Source: CAD feature listing. Evaluate the final solid. Frame: model axes, mm. Face numbers are marked on the shaded views. A direction names the side the tool comes from. Give positions to 0.01 mm unless a question says otherwise; leave off trailing zeros. Order: outer loops, then holes, each group sorted by start corner. A loop starts at its lowest first (then second) coordinate and runs counter-clockwise, first axis right, second up. Notation, with made-up numbers: M -9,69.25 L 38,69.25 A15 cw 38,84.25 Z; hole C 66,-38.5 d9. An arc over 180 degrees is marked long. Answer as a JSON object with one key per item and string values. Group by question number.
1. Section query D-D (x = -21). Output: boundary loops of the cut face in (y, z), plus the area to 3 significant figures.
2. Set-up query: the marked faces 4, 5 and 6. Return all of +Z, -Z, +X, -X, +Y, -Y with unobstructed straight access to the full face (end or side cutting, diameter ignored); none if empty.
3. Section query C-C (z = 5.25). Output: boundary loops of the cut face in (x, y), plus the area to 3 significant figures.
4. Pin query (flat end, axial travel): P1, Ø1.5, axis at x = -25.5, y = -0.5, coming from the +Z side; P2, Ø2, axis at x = 10.5, z = 3.5, coming from the -Y side; P3, Ø15.5, axis at x = 12, y = -11, coming from the -Z side; P4, Ø4.5, axis at x = 11.5, y = 17.5, coming from the +Z side. Return the tip coordinate at first contact, or that it passes through.
5. Pull-direction query (Y, two-part tool) for the marked faces 1, 2 and 3; classes: +Y half, -Y half, draft (parallel to the pull), parting line (faces both ways), or undercut.
6. Section query B-B (x = 10.5). Output: boundary loops of the cut face in (y, z).
7. Section query A-A (y = 12.5). Output: boundary loops of the cut face in (x, z), plus the area to 3 significant figures.
8. Material intervals for L1, parallel to Y at x = 0, z = -2.5; L2, parallel to X at y = -10, z = -2; L3, parallel to Y at x = 0, z = -4.5, sorted ascending. Write a range as [from, to].
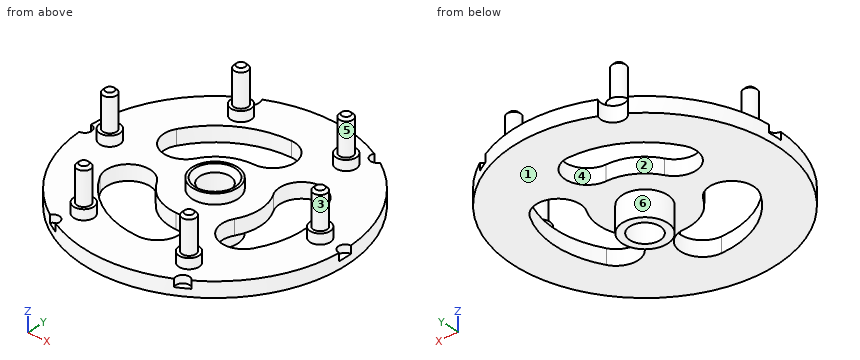
from build123d import *

# Parameters (mm, degrees)
SKETCH_1_R               = 26
EXTRUDE_1_DEPTH          = 3
SKETCH_2_R               = 1.35
EXTRUDE_2_DEPTH          = 9
SKETCH_4_R               = 2
EXTRUDE_4_DEPTH          = 2
SKETCH_5_R               = 3
CUT_EXTRUDE_1_DEPTH      = 38.854986461
SKETCH_7_R               = 4.5
SKETCH_7_R_2             = 3
EXTRUDE_1_2_DEPTH        = 8
EXTRUDE_START            = 2
SKETCH_8_R               = 4.5
SKETCH_8_R_2             = 3
EXTRUDE_2_2_DEPTH        = 2
CUT_EXTRUDE_2_REACH      = 39.855
SKETCH_9_R               = 2.326383569
SKETCH_10_R              = 1.343821969
CUT_EXTRUDE_3_DEPTH      = 1.5
CUT_EXTRUDE_4_REACH      = 40.678
CHAMFER_1_SIZE           = 1
CHAMFER_3_SIZE           = 0.5
PATTERN_CIRCULAR_1_COUNT = 3


with BuildPart() as part:
    # Sketch 1 → Extrude 1 (new body)
    with BuildSketch(Plane.XY):
        Circle(SKETCH_1_R)
    extrude(amount=-EXTRUDE_1_DEPTH)

    # Sketch 2 → Extrude 2 (add)
    with BuildSketch(Plane.XY):
        with Locations((-21, 0)):
            Circle(SKETCH_2_R)
        with Locations((-10.5, 18.186533479)):
            Circle(SKETCH_2_R)
        with Locations((10.5, 18.186533479)):
            Circle(SKETCH_2_R)
        with Locations((21, 0)):
            Circle(SKETCH_2_R)
        with Locations((10.5, -18.186533479)):
            Circle(SKETCH_2_R)
        with Locations((-10.5, -18.186533479)):
            Circle(SKETCH_2_R)
    extrude(amount=EXTRUDE_2_DEPTH)

    # Sketch 4 → Extrude 4 (add)
    with BuildSketch(Plane.XY):
        with Locations((-10.5, 18.186533479)):
            Circle(SKETCH_4_R)
        with Locations((10.5, 18.186533479)):
            Circle(SKETCH_4_R)
        with Locations((21, 0)):
            Circle(SKETCH_4_R)
        with Locations((10.5, -18.186533479)):
            Circle(SKETCH_4_R)
        with Locations((-10.5, -18.186533479)):
            Circle(SKETCH_4_R)
        with Locations((-21, 0)):
            Circle(SKETCH_4_R)
    extrude(amount=EXTRUDE_4_DEPTH)

    # Sketch 5 → Cut-Extrude 1 (cut, through all)
    with BuildSketch(Plane.XY):
        Circle(SKETCH_5_R)
    extrude(amount=-CUT_EXTRUDE_1_DEPTH, mode=Mode.SUBTRACT)

    # Sketch 7 → Extrude 1 2 (add)
    with BuildSketch(Plane.XY):
        Circle(SKETCH_7_R)
        Circle(SKETCH_7_R_2, mode=Mode.SUBTRACT)
    extrude(amount=-EXTRUDE_1_2_DEPTH)

    # Sketch 8 → Extrude 2 2 (add)
    with BuildSketch(Plane.XY.offset(EXTRUDE_START)):
        Circle(SKETCH_8_R)
        Circle(SKETCH_8_R_2, mode=Mode.SUBTRACT)
    extrude(amount=-EXTRUDE_2_2_DEPTH)

    # Sketch 9 → Cut-Extrude 2 (cut, up to next)
    with BuildSketch(Plane.XY, mode=Mode.PRIVATE) as cut_extrude_2_sk1:
        with Locations((-13, 22.516660498)):
            Circle(SKETCH_9_R)
    cut_extrude_2_tool1 = extrude(cut_extrude_2_sk1.sketch, amount=-CUT_EXTRUDE_2_REACH, mode=Mode.PRIVATE) & part.part
    add(cut_extrude_2_tool1.solids().sort_by_distance((-13, 22.51666, 0))[0], mode=Mode.SUBTRACT)

    # Sketch 10 → Cut-Extrude 3 (cut)
    with BuildSketch(Plane.XY):
        with Locations((-13, 22.516660498)):
            Circle(SKETCH_10_R)
        with Locations((13, 22.516660498)):
            Circle(SKETCH_10_R)
        with Locations((26, 0)):
            Circle(SKETCH_10_R)
        with Locations((13, -22.516660498)):
            Circle(SKETCH_10_R)
        with Locations((-13, -22.516660498)):
            Circle(SKETCH_10_R)
        with Locations((-26, 0)):
            Circle(SKETCH_10_R)
    extrude(amount=-CUT_EXTRUDE_3_DEPTH, mode=Mode.SUBTRACT)

    # Sketch 11 → Cut-Extrude 4 (cut, up to next)
    with BuildSketch(Plane(origin=(0, 0, -3), x_dir=(-1, 0, 0), z_dir=(0, 0, -1)), mode=Mode.PRIVATE) as cut_extrude_4_sk1:
        with BuildLine():
            ThreePointArc((15.338641918, 8.855769041), (8.855769041, 15.338641918), (0, 17.711538081))
            ThreePointArc((0, 17.711538081), (-4.370103516, 13.341434566), (0, 8.97133105))
            ThreePointArc((0, 8.97133105), (4.485665525, 7.769400595), (7.769400595, 4.485665525))
            ThreePointArc((7.769400595, 4.485665525), (13.739073015, 2.886096621), (15.338641918, 8.855769041))
        make_face()
    cut_extrude_4_tool1 = extrude(cut_extrude_4_sk1.sketch, amount=-CUT_EXTRUDE_4_REACH, mode=Mode.PRIVATE) & part.part
    cut_extrude_4 = cut_extrude_4_tool1.solids().sort_by_distance((-6.174677, 10.694854, -3))[0]
    add(cut_extrude_4, mode=Mode.SUBTRACT)

    # Chamfer 1
    chamfer_1_edges = [part.edges().sort_by_distance(p)[0] for p in [
        (-3, 0, 2),
    ]]
    chamfer(chamfer_1_edges, length=CHAMFER_1_SIZE)

    # Chamfer 3
    chamfer_3_edges = [part.edges().sort_by_distance(p)[0] for p in [
        (-11.85, 18.186533479, 9),
        (9.15, 18.186533479, 9),
        (19.65, 0, 9),
        (9.15, -18.186533479, 9),
        (-11.85, -18.186533479, 9),
        (-22.35, 0, 9),
    ]]
    chamfer(chamfer_3_edges, length=CHAMFER_3_SIZE)

    # Pattern Circular 1: Cut-Extrude 4 ×3 about axis
    pattern_circular_1_axis = Axis((0, 0, 0), (0, 0, 1))
    for i in range(1, PATTERN_CIRCULAR_1_COUNT):
        add(cut_extrude_4.rotate(pattern_circular_1_axis, i * 360 / PATTERN_CIRCULAR_1_COUNT), mode=Mode.SUBTRACT)


solid = part.part
Answer sheet:
{
 "1": {"outline": "M -15.33,-3 L 15.33,-3 L 15.33,0 L 2,0 L 2,2 L 1.35,2 L 1.35,8.5 L 0.85,9 L -0.85,9 L -1.35,8.5 L -1.35,2 L -2,2 L -2,0 L -15.33,0 Z", "area": "119 mm^2"},
 "2": {"face 4": "+Z, -Z", "face 5": "+Z", "face 6": "-Z"},
 "3": {"outline": "C -21,0 d2.7; C -10.5,-18.19 d2.7; C -10.5,18.19 d2.7; C 10.5,-18.19 d2.7; C 10.5,18.19 d2.7; C 21,0 d2.7", "area": "34.4 mm^2"},
 "4": {"P1": "z = 0", "P2": "y = -19.54", "P3": "z = -3", "P4": "z = 9"},
 "5": {"face 1": "draft", "face 2": "undercut", "face 3": "parting line"},
 "6": {"outline": "M -23.79,-3 L -10.91,-3 L -10.91,0 L -16.19,0 L -16.19,2 L -16.84,2 L -16.84,8.5 L -17.34,9 L -19.04,9 L -19.54,8.5 L -19.54,2 L -20.19,2 L -20.19,0 L -23.79,0 Z; M 10.91,-3 L 23.79,-3 L 23.79,0 L 20.19,0 L 20.19,2 L 19.54,2 L 19.54,8.5 L 19.04,9 L 17.34,9 L 16.84,8.5 L 16.84,2 L 16.19,2 L 16.19,0 L 10.91,0 Z"},
 "7": {"outline": "M -22.8,-3 L -12.55,-3 L -12.55,0 L -22.8,0 Z; M 4.29,-3 L 22.8,-3 L 22.8,0 L 4.29,0 Z", "area": "86.3 mm^2"},
 "8": {"L1": "[-26, -17.71], [-8.97, -3], [3, 8.97], [17.71, 26]", "L2": "[-24, -14.62], [2.82, 8.72], [14.38, 24]", "L3": "[-4.5, -3], [3, 4.5]"}
}
